Design review of the part built by this model. Coordinates are the model's own, in mm. A direction names the side the tool comes from. Round coordinates to 2 decimals unless told otherwise and drop trailing zeros. Order: outer loops, then holes, each group sorted by start corner. A loop starts at its lowest first (then second) coordinate and runs counter-clockwise, first axis right, second up. Notation, with made-up numbers: (-38, -38.5) - (7, -38.5) arc R20 ccw to (7, -20.5) - close; hole circle Ø9 at (39, 20.25). An arc over 180 degrees is marked (long way). Use CSV: the item, a comma, the result in double quotes. Start each with the question number.
Autodesk Inventor part; units mm, degrees
ref_plane "YZ Plane" through (0, 0, 0) normal (1, 0, 0) x (0, 1, 0)
ref_plane "XZ Plane" through (0, 0, 0) normal (0, 1, 0) x (-1, 0, 0)
ref_plane "XY Plane" through (0, 0, 0) normal (0, 0, 1) x (1, 0, 0)
sketch "スケッチ1" plane through (0, 0, 0) normal (1, 0, 0) x (0, 1, 0)
  line L0 (-65.2534, -641.9406) -> (-65.2534, 666.0594)
  line L1 (-65.2534, -539.9406) -> (339.7466, -539.9406)
  line L2 (339.7466, -539.9406) -> (339.7466, -519.9406)
  line L3 (339.7466, -519.9406) -> (-65.2534, -519.9406)
  line L4 (-65.2534, -519.9406) -> (-65.2534, -539.9406)
  circle A0 centre (-30.0734, -492.9406) radius 21
  circle A1 centre (-30.0734, -450.9406) radius 16
  circle A2 centre (-30.0734, -450.9406) radius 13.68
  line L5 (-85.2534, -641.9406) -> (-65.2534, -641.9406)
  line L6 (-85.2534, -641.9406) -> (-65.2534, -641.9406)
  line L7 (-85.2534, -641.9406) -> (398.7466, -641.9406)
  line L8 (398.7466, -641.9406) -> (398.7466, -661.9406)
  line L9 (398.7466, -661.9406) -> (-85.2534, -661.9406)
  line L10 (-85.2534, -661.9406) -> (-85.2534, -641.9406)
  line L11 (-10.0734, 666.0594) -> (9.1023, 671.742)
  line L12 (9.1023, 671.742) -> (394.9497, -630.2894)
  line L13 (394.9497, -630.2894) -> (375.774, -635.972)
  line L14 (375.774, -635.972) -> (-10.0734, 666.0594)
  line L15 (-85.2534, 666.0594) -> (-85.2534, -641.9406)
  line L16 (-85.2534, -434.9406) -> (-30.0734, -434.9406)
  line L17 (-9.0734, -492.9406) -> (-9.0734, -539.9406)
  line L18 (-9.0734, -492.9406) -> (-9.0734, -434.9406)
  line L19 (-9.0734, -434.9406) -> (-30.0734, -434.9406)
  circle A3 centre (-75.2534, -446.9406) radius 1.5
  circle A4 centre (-75.2534, -456.9406) radius 1.5
  line L20 (-30.0734, -466.9406) -> (-85.2534, -466.9406)
  circle A5 centre (-55.2534, -529.9406) radius 1.5
  circle A6 centre (-35.2534, -529.9406) radius 1.5
  line L21 (-65.2534, -539.9406) -> (-85.2534, -539.9406)
  circle A7 centre (-75.2534, -529.9406) radius 1.5
  circle A8 centre (-75.2534, -509.9406) radius 1.5
  circle A9 centre (-30.0734, 650.0594) radius 16
  line L22 (-65.2534, 666.0594) -> (-85.2534, 666.0594)
  line L23 (-85.2534, 666.0594) -> (-30.0734, 666.0594)
  line L24 (-30.0734, 634.0594) -> (-85.2534, 634.0594)
  line L25 (-30.0734, 666.0594) -> (-10.0734, 666.0594)
  circle A10 centre (-30.0734, 650.0594) radius 7.5
  line L26 (-30.0734, 634.0594) -> (-0.5904, 634.0594)
  circle A11 centre (-75.2534, 654.0594) radius 1.5
  circle A12 centre (-75.2534, 644.0594) radius 1.5
  circle A13 centre (2.3558, 659.3128) radius 1.5
  circle A14 centre (5.1971, 649.725) radius 1.5
  line L27 (-0.5904, 634.0594) -> (18.5853, 639.742)
  line L28 (-65.2534, -601.9406) -> (-45.2534, -641.9406)
  line L29 (-45.2534, -641.9406) -> (-45.2534, -661.9406)
  line L30 (-65.2534, -601.9406) -> (-85.2534, -601.9406)
  circle A15 centre (-75.2534, -631.9406) radius 1.5
  circle A16 centre (-75.2534, -621.9406) radius 1.5
  circle A17 centre (-75.2534, -611.9406) radius 1.5
  circle A18 centre (-75.2534, -651.9406) radius 1.5
  circle A19 centre (-65.2534, -651.9406) radius 1.5
  circle A20 centre (-55.2534, -651.9406) radius 1.5
  line L31 (-85.2534, -641.9406) -> (-85.2534, -601.9406)
  line L32 (368.7466, -641.9406) -> (368.7466, -661.9406)
  line L33 (367.2501, -607.2084) -> (386.4258, -601.5259)
  line L34 (375.774, -635.972) -> (377.5427, -641.9406)
  line L35 (394.9497, -630.2894) -> (398.7466, -641.9406)
  circle A21 centre (378.7466, -651.9406) radius 1.5
  circle A22 centre (388.7466, -651.9406) radius 1.5
  circle A23 centre (382.5205, -623.5429) radius 1.5
  circle A24 centre (379.6792, -613.955) radius 1.5
  circle A25 centre (319.7466, -529.9406) radius 1.5
  circle A26 centre (329.7466, -529.9406) radius 1.5
  line L36 (339.7466, -519.9406) -> (341.3889, -519.9406)
  line L37 (339.7466, -539.9406) -> (347.3158, -539.9406)
  line L38 (341.3889, -519.9406) -> (362.2486, -519.9406)
  circle A27 centre (354.6759, -529.5818) radius 1.5
  circle A28 centre (357.5172, -539.1697) radius 1.5
  line L39 (350.7706, -551.5989) -> (369.9463, -545.9163)
  line L40 (309.7466, -519.9406) -> (309.7466, -539.9406)
  point P0 (0, 0)
  point P1 (-388.2534, -209.6072)
  point P2 (-65.2534, -519.9406)
  point P3 (385.3618, -633.1307)
  dimension "d1" = 42
  dimension "d0" = 20
  dimension "d2" = 32
  dimension "d3" = 27.36
  dimension "d4" = 35.18
  dimension "d5" = 35.18
  dimension "d6" = 27
  dimension "d7" = 42
  dimension "d8" = 191
  dimension "d9" = 20
  dimension "d10" = 484
  dimension "d11" = 3
  dimension "d12" = 3
  dimension "d13" = 10
  dimension "d14" = 10
  dimension "d15" = 10
  dimension "d16" = 10
  dimension "d17" = 3
  dimension "d18" = 3
  dimension "d19" = 10
  dimension "d20" = 20
  dimension "d21" = 10
  dimension "d22" = 10
  dimension "d23" = 3
  dimension "d24" = 3
  dimension "d25" = 10
  dimension "d26" = 20
  dimension "d27" = 10
  dimension "d28" = 10
  dimension "d29" = 20
  dimension "d30" = 32
  dimension "d31" = 35.18
  dimension "d32" = 20
  dimension "d33" = 1358
  dimension "d34" = 91.543
  dimension "d35" = 405
  dimension "d36" = 15
  dimension "d37" = 3
  dimension "d38" = 3
  dimension "d39" = 10
  dimension "d40" = 10
  dimension "d41" = 10
  dimension "d42" = 10
  dimension "d43" = 3
  dimension "d44" = 3
  dimension "d45" = 10
  dimension "d46" = 10
  dimension "d47" = 10
  dimension "d48" = 10
  dimension "d49" = 40
  dimension "d50" = 3
  dimension "d51" = 3
  dimension "d52" = 3
  dimension "d53" = 3
  dimension "d54" = 3
  dimension "d55" = 3
  dimension "d56" = 10
  dimension "d57" = 10
  dimension "d58" = 10
  dimension "d59" = 10
  dimension "d60" = 10
  dimension "d61" = 10
  dimension "d62" = 10
  dimension "d63" = 10
  dimension "d64" = 10
extrude "押し出し1" add sketch "スケッチ1" against normal blind 2 contours L40 L3 L2 L1 | L2 L36 L14 L37 | L14 L38 L12 L39
fillet "フィレット1" radius 2 6 edges at (-1, 309.7466, -519.9406) (-1, 309.7466, -539.9406) (-1, 347.3158, -539.9406) (-1, 350.7706, -551.5989) (-1, 369.9463, -545.9163) (-1, 362.2486, -519.9406)
equation "\"d14\" = d15"
equation "\"d21\" = d19"
equation "\"d22\" = d19"
equation "\"d27\" = d25"
equation "\"d28\" = d25"
equation "\"d31\" = d4"
equation "\"d41\" = d39"
equation "\"d42\" = d39"
equation "\"d46\" = d45"
equation "\"d47\" = d45"
equation "\"d48\" = d45"
equation "\"d57\" = d56"
equation "\"d58\" = d56"
equation "\"d59\" = d56"
equation "\"d60\" = d56"
equation "\"d61\" = d56"
equation "\"d62\" = d56"
equation "\"d63\" = d56"
equation "\"d64\" = d62"
properties part number "dribl-v1-Plate-11" material "アルミニウム 6061"
Q1. Take a section at C-C (y = 344). State the section outline as (x, z) points, plus the area to 3 significant figures.
Q2. Take a section at A-A (x = -1.3). State the section outline as (y, z) points, plus the area to 3 significant figures.
Q3. Tool access review of faces 1 (the flat face through (-0.99, 360.25, -548.79)), 2 (the flat face through (-1, 329, -539.941)): name each direction out of +Z, -Z, +X, -X, +Y, -Y from which nothing blocks a thin tool from reaching the whole face with its end or side.
Q4. Take a section at B-B (z = -530.5). State the section outline as (x, y) points, plus the area to 3 significant figures.
Q5. The part is to be moulded in two halves that separate along Z. For faces 3 (the flat face through (0, 339, -532)), 4 (the cylindrical face through (-0.99, 355.37, -530.91)), 5 (the flat face through (-0.99, 365.98, -532.53)), say which applies: +Z half, -Z half, draft (parallel to the pull), parting line (faces both ways), or undercut.
Q6. Take a section at D-D (z = -548). State the section outline as (x, y) points.
Q7. For L1, parallel to Z at x = -0.55, y = 342.5; L2, parallel to Y at x = -0.2, z = -530.5; L3, parallel to Z at x = -1.1, y = 354, list the stretches that pass through material, from the lowest coordinate up. Write a range as [from, to].
Findings below:
1,outline,"(-2, -539.94) - (0, -539.94) - (0, -519.94) - (-2, -519.94) - close"
1,area,"40.0 mm^2"
2,outline,"(309.75, -537.94) arc R2 ccw to (311.75, -539.94) - (345.82, -539.94) arc R2 cw to (347.74, -541.37) - (350.2, -549.68) arc R2 ccw to (352.69, -551.03) - (368.03, -546.48) arc R2 ccw to (369.38, -544) - (362.67, -521.37) arc R2 ccw to (360.76, -519.94) - (311.75, -519.94) arc R2 ccw to (309.75, -521.94) - close; hole circle Ø3 at (319.75, -529.94); hole circle Ø3 at (329.75, -529.94); hole circle Ø3 at (354.68, -529.58); hole circle Ø3 at (357.52, -539.17)"
2,area,"1,260 mm^2"
3,face 1,"-Z, +X, -X, +Y"
3,face 2,"-Z, +X, -X, -Y"
4,outline,"(-2, 309.75) - (0, 309.75) - (0, 318.35) - (-2, 318.35) - close; (-2, 321.14) - (0, 321.14) - (0, 328.35) - (-2, 328.35) - close; (-2, 331.14) - (0, 331.14) - (0, 353.49) - (-2, 353.49) - close; (-2, 355.86) - (0, 355.86) - (0, 365.38) - (-2, 365.38) - close"
4,area,"95.4 mm^2"
5,face 3,"draft"
5,face 4,"undercut"
5,face 5,"+Z half"
6,outline,"(-2, 349.7) - (0, 349.7) - (0, 362.91) - (-2, 362.91) - close"
7,L1,"z = [-539.94, -519.94]"
7,L2,"y = [309.75, 318.35], [321.14, 328.35], [331.14, 353.49], [355.86, 365.38]"
7,L3,"z = [-550.64, -530.92], [-528.24, -519.94]"
